```python
from build123d import *

# Parameters (mm, degrees)
SKETCH1_W           = 125
SKETCH1_H           = 25
SKETCH1_W_2         = 10.0584
SKETCH1_H_2         = 10.0584
SKETCH1_W_3         = 52.8
SKETCH1_H_3         = 20
SKETCH1_H_4         = 7.6454
SKETCH1_R           = 1.5
SKETCH1_W_4         = 6.588
SKETCH1_H_5         = 9.25
SKETCH1_R_2         = 2.25
BOSS_EXTRUDE1_DEPTH = 5
SKETCH3_W           = 125
SKETCH3_H           = 8
BOSS_EXTRUDE2_DEPTH = 2
BOSS_EXTRUDE3_START = -25
SKETCH3_2_W         = 125
SKETCH3_2_H         = 8
BOSS_EXTRUDE3_DEPTH = 2


with BuildPart() as part:
    # Sketch1 → Boss-Extrude1 (new body)
    with BuildSketch(Plane.XY):
        Rectangle(SKETCH1_W, SKETCH1_H)
        with Locations((-47.5, 0)):
            Rectangle(SKETCH1_W_2, SKETCH1_H_2, mode=Mode.SUBTRACT)
        with Locations((33.1, 0)):
            Rectangle(SKETCH1_W_3, SKETCH1_H_3, mode=Mode.SUBTRACT)
        with Locations((-47.5, 0)):
            Rectangle(SKETCH1_W_2, SKETCH1_H_4)
        with Locations((-47.5, 0)):
            Circle(SKETCH1_R, mode=Mode.SUBTRACT)
        with Locations((56.206, 5.375)):
            Rectangle(SKETCH1_W_4, SKETCH1_H_5)
        with Locations((57, 5.1)):
            Circle(SKETCH1_R_2, mode=Mode.SUBTRACT)
        with Locations((56.206, -5.375)):
            Rectangle(SKETCH1_W_4, SKETCH1_H_5)
        with Locations((57, -5.1)):
            Circle(SKETCH1_R_2, mode=Mode.SUBTRACT)
        with Locations((9.994, -5.375)):
            Rectangle(SKETCH1_W_4, SKETCH1_H_5)
        with Locations((9.2, -5.1)):
            Circle(SKETCH1_R_2, mode=Mode.SUBTRACT)
        with Locations((9.994, 5.375)):
            Rectangle(SKETCH1_W_4, SKETCH1_H_5)
        with Locations((9.2, 5.1)):
            Circle(SKETCH1_R_2, mode=Mode.SUBTRACT)
    extrude(amount=BOSS_EXTRUDE1_DEPTH)

    # Sketch3 → Boss-Extrude2 (add)
    with BuildSketch(Plane(origin=(0, 12.5, 0), x_dir=(1, 0, 0), z_dir=(0, 1, 0))):
        with Locations((0, -1)):
            Rectangle(SKETCH3_W, SKETCH3_H)
    extrude(amount=-BOSS_EXTRUDE2_DEPTH)

    # Sketch3<2> → Boss-Extrude3 (add)
    with BuildSketch(Plane(origin=(0, 12.5, 0), x_dir=(1, 0, 0), z_dir=(0, 1, 0)).offset(BOSS_EXTRUDE3_START)):
        with Locations((0, -1)):
            Rectangle(SKETCH3_2_W, SKETCH3_2_H)
    extrude(amount=BOSS_EXTRUDE3_DEPTH)


solid = part.part
```
Design review of the part built by this model. Coordinates are the model's own, in mm. A direction names the side the tool comes from. Give positions to 0.01 mm unless a question says otherwise; leave off trailing zeros. Order: outer loops, then holes, each group sorted by start corner. A loop starts at its lowest first (then second) coordinate and runs counter-clockwise, first axis right, second up. Notation, with made-up numbers: (66.5, -18) -> (121.5, -18) arc R25 cw to (121.5, 13) -> close; hole circle Ø4 at (10, -17). An arc over 180 degrees is marked (long way). Write item = value, one per line. Start each with the question number.
(1) We need section A-A on x = 57. Write out the cut boundary in (y, z).
(2) We need section C-C on x = -34. Write out the cut boundary in (y, z), plus the area to 3 significant figures.
(3) Mouldability with a two-part tool opening along X and no side actions: class faces 1 (the face through (-62.5, 0, 2)), 2 (the face through (56, 0.75, 2)), 3 (the face through (-1, -10.5, -2)) as +X half, -X half, draft (parallel to the pull), parting line (faces both ways), or undercut.
(4) To check wall thickness, follow line 1 along Y through (x, z) = (57, 3.95); line 2 along Y through (x, z) = (46, -0.5); line 3 along X through (y, z) = (6.25, 3.5). State the ranges of each line that lie inside material, in increasing order.
(5) We need section B-B on z = 3.25. State how many separate pieces and enclosed holes the cut face has, plus the area to 3 significant figures.
(6) For faces 4 (the face through (-1, 12.5, 1)), 5 (the face through (-15, 0, 0)), 6 (the face through (-48, -5.029, 2)), list the 3-axis set-ups (+Z, -Z, +X, -X, +Y, -Y) from which the entire face can be reached by the end or side of a thin tool; tool diameter is ignored.
(7) For pin 1 (3.5 mm diameter, centred on x = 9.2, y = -5.1, fed in from +Z), flat-tipped, find the tip position at first contact; note if it passes through.
(8) We need section D-D on x = -47.5. Write out the cut boundary in (y, z).
Numbers:
q1.outline = (-12.5, -3) -> (-10.5, -3) -> (-10.5, 0) -> (-7.35, 0) -> (-7.35, 5) -> (-12.5, 5) -> close; (-2.85, 0) -> (-0.75, 0) -> (-0.75, 5) -> (-2.85, 5) -> close; (0.75, 0) -> (2.85, 0) -> (2.85, 5) -> (0.75, 5) -> close; (7.35, 0) -> (10.5, 0) -> (10.5, -3) -> (12.5, -3) -> (12.5, 5) -> (7.35, 5) -> close
q2.outline = (-12.5, -3) -> (-10.5, -3) -> (-10.5, 0) -> (10.5, 0) -> (10.5, -3) -> (12.5, -3) -> (12.5, 5) -> (-12.5, 5) -> close
q2.area = 137 mm^2
q3.face_1 = -X half
q3.face_2 = undercut
q3.face_3 = draft
q4.line_1 = -12.5 to -7.35, -2.85 to -0.75, 0.75 to 2.85, 7.35 to 12.5
q4.line_2 = -12.5 to -10.5, 10.5 to 12.5
q4.line_3 = -62.5 to 7.27, 11.13 to 13.29, 52.91 to 55.07, 58.93 to 62.5
q5.separate_pieces = 1
q5.enclosed_holes = 8
q5.area = 2,220 mm^2
q6.face_4 = +Z, -Z, +X, -X, +Y
q6.face_5 = -Z, +X, -X
q6.face_6 = +Z, -Z
q7.pin_1 = through
q8.outline = (-12.5, -3) -> (-10.5, -3) -> (-10.5, 0) -> (-5.03, 0) -> (-5.03, 5) -> (-12.5, 5) -> close; (-3.82, 0) -> (-1.5, 0) -> (-1.5, 5) -> (-3.82, 5) -> close; (1.5, 0) -> (3.82, 0) -> (3.82, 5) -> (1.5, 5) -> close; (5.03, 0) -> (10.5, 0) -> (10.5, -3) -> (12.5, -3) -> (12.5, 5) -> (5.03, 5) -> close
